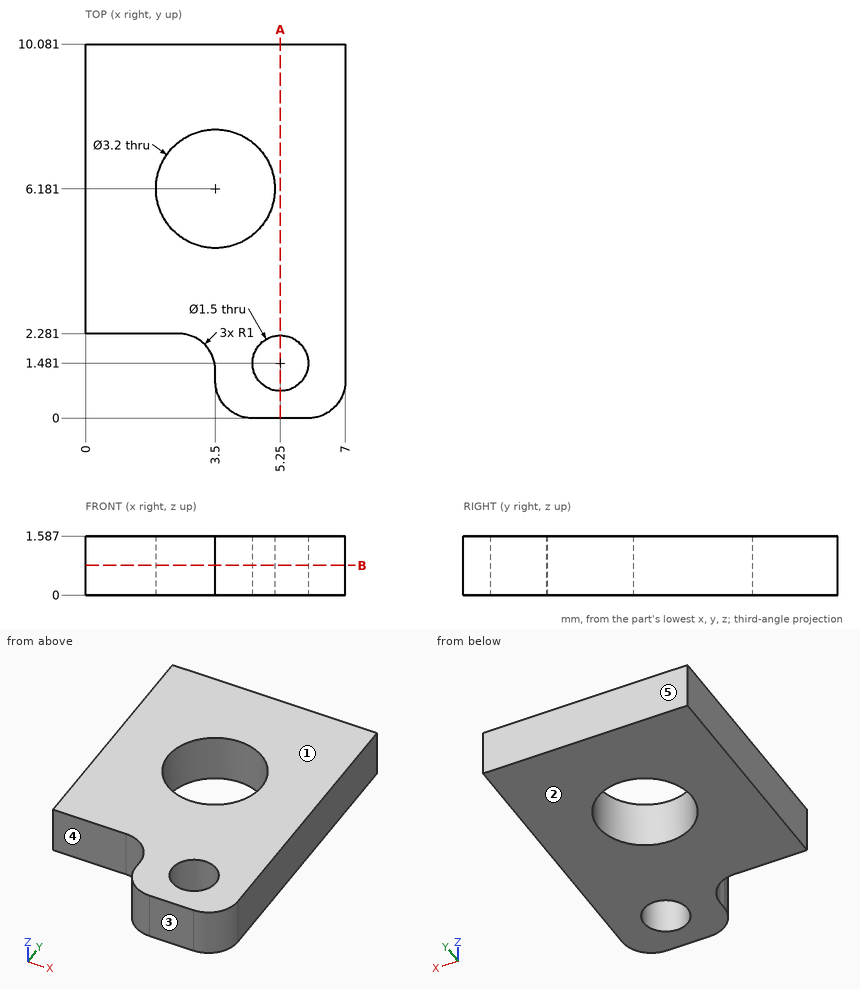
The drawing under review shows one solid part. Ordinate dimensions are in mm from its lowest x, y, z. A direction names the side the tool comes from. Give positions to 0.01 mm unless a question says otherwise; leave off trailing zeros. Write each loop counter-clockwise with the first axis right and the second up, starting at its lowest first coordinate (ties: lowest second). Pieces come first, ordered by that corner, then holes. Notation, with made-up numbers: (31.5, 72.25) - (37.5, 72.25) arc R5 cw to (37.5, 78.25) - close; hole circle Ø1 at (-4, 12.5). An arc over 180 degrees is marked (long way). Answer in a Markdown table with one row per item. Add a question column.
1. Tool access review of the marked faces 4 and 5: name each direction out of +Z, -Z, +X, -X, +Y, -Y from which nothing blocks a thin tool from reaching the whole face with its end or side.
2. Insertion check: P1, Ø0.5, axis at x = 1, z = 0.5, coming from the -Y side. The pin has a flat end and moves straight along its axis. Give the tip position at first contact, or say it passes through.
3. Draft analysis for pull direction Z (two halves, no side actions). For the marked faces 1, 2 and 3, state which applies: +Z half, -Z half, draft (parallel to the pull), parting line (faces both ways), or undercut.
4. Wall thickness on line 1 along Y through (x, z) = (5.25, 1); line 2 along X through (y, z) = (5.75, 1.55); line 3 along X through (y, z) = (1.5, 0.75) (1 decimal): over which ranges is each line inside the solid? List them lowest first. Write a range as [from, to].
5. We need section B-B on z = 0.8. Write out the cut boundary in (x, y).
6. We need section A-A on x = 5.25. Write out the cut boundary in (y, z), then the cut area to 3 significant figures.
Ans:
| question | item | result |
|---|---|---|
| 1 | face 4 | +Z, -Z, -X, -Y |
| 1 | face 5 | +Z, -Z, +X, -X, +Y |
| 2 | P1 | stops at y = 2.28 |
| 3 | face 1 | +Z half |
| 3 | face 2 | -Z half |
| 3 | face 3 | draft |
| 4 | line 1 | y = [0, 0.73], [2.23, 10.08] |
| 4 | line 2 | x = [0, 1.96], [5.04, 7] |
| 4 | line 3 | x = [3.5, 4.5], [6, 7] |
| 5 | outline | (0, 2.28) - (2.5, 2.28) arc R1 cw to (3.5, 1.28) - (3.5, 1) arc R1 ccw to (4.5, 0) - (6, 0) arc R1 ccw to (7, 1) - (7, 10.08) - (0, 10.08) - close; hole circle Ø3.2 at (3.5, 6.18); hole circle Ø1.5 at (5.25, 1.48) |
| 6 | outline | (0, 0) - (0.73, 0) - (0.73, 1.59) - (0, 1.59) - close; (2.23, 0) - (10.08, 0) - (10.08, 1.59) - (2.23, 1.59) - close |
| 6 | area | 13.6 mm^2 |
